Input: dimensioned drawing with shaded views. Units: mm. Origin: part minimum x, y, z. A direction names the side the tool comes from. Round coordinates to 2 decimals unless told otherwise and drop trailing zeros. Loops run counter-clockwise (first coordinate to the right, second up) from the corner with the lowest first, then second, coordinate; pieces in that order, holes last. Notation, with made-up numbers: (14.5, 26.5) - (27.5, 26.5) arc R21 cw to (27.5, 53.5) - close; hole circle Ø2 at (-20.75, -32.5). An arc over 180 degrees is marked (long way). One line per question, with ' | ' between items.
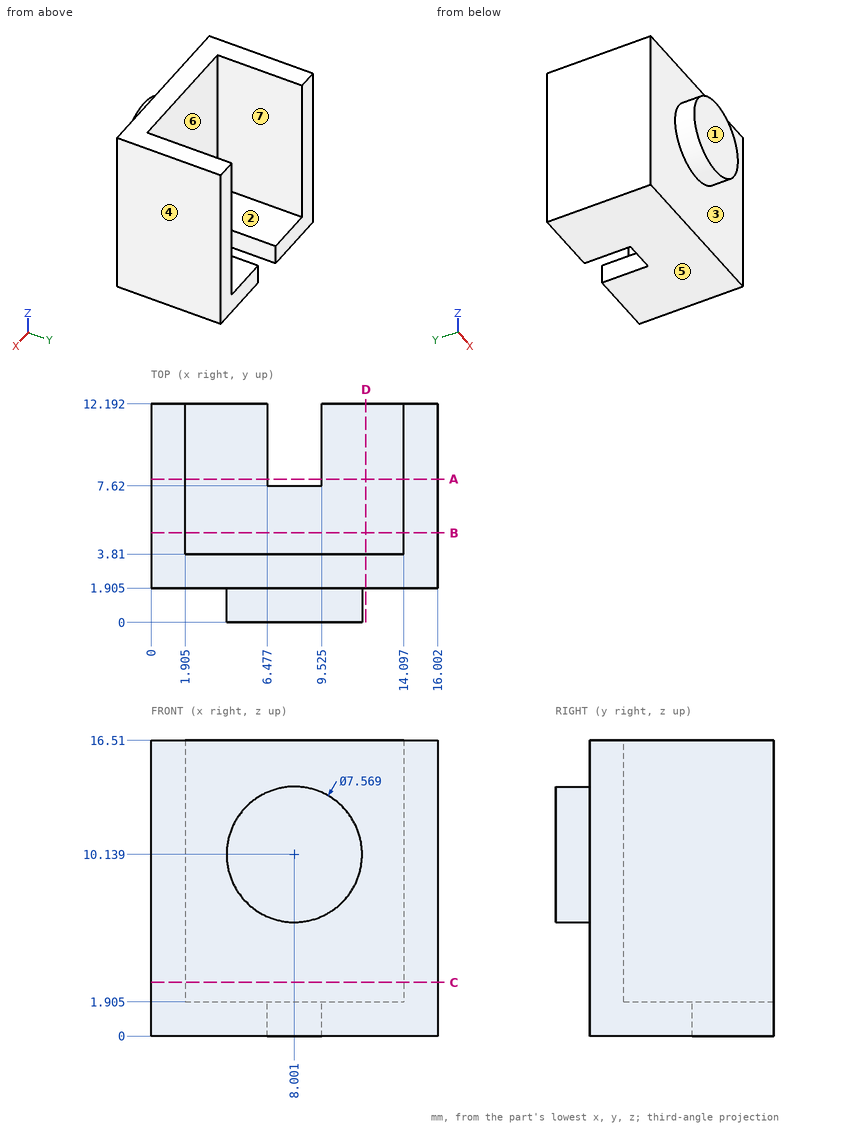
1. Material intervals for probe 1 along X at (y, z) = (9, 7) (1 decimal); probe 2 along Z at (x, y) = (5.5, 7) (1 decimal); probe 3 along Y at (x, z) = (5.5, 12.5), sorted ascending.
Worked out:
probe 1: x = 0 to 1.9, 14.1 to 16 | probe 2: z = 0 to 1.9 | probe 3: y = 0 to 3.81
2. Contact query for flat-ended pins moving along their axis: P1, Ø5, axis at x = 8, z = 8, coming from the +Y side; P2, Ø1.5, axis at x = 8.5, z = 1.5, coming from the +Y side; P3, Ø6.5, axis at x = 7, y = 9, coming from the +Z side (3 decimals). Output: stop coordinate, or through.
Worked out:
P1: stops at y = 3.81 | P2: stops at y = 7.62 | P3: stops at z = 1.905
3. Section query C-C, the plane z = 3. Return loops of the section in (x, y) (1 decimal).
Worked out:
outline: (0, 1.9) - (16, 1.9) - (16, 12.2) - (14.1, 12.2) - (14.1, 3.8) - (1.9, 3.8) - (1.9, 12.2) - (0, 12.2) - close
4. Access query for the marked faces 1, 2 and 3. Directions: +Z, -Z, +X, -X, +Y, -Y. A direction counts if a zero-diameter tool reaches every point of the face in a straight line with its end or side. Return the directions, or none.
Worked out:
face 1: +Z, -Z, +X, -X, -Y | face 2: +Z, +Y | face 3: -Y
5. Section query D-D, the plane x = 12. Return loops of the section in (y, z) (1 decimal).
Worked out:
outline: (1.9, 0) - (12.2, 0) - (12.2, 1.9) - (3.8, 1.9) - (3.8, 16.5) - (1.9, 16.5) - close
6. Section query B-B, the plane y = 5. Return loops of the section in (x, z) (1 decimal).
Worked out:
outline: (0, 0) - (16, 0) - (16, 16.5) - (14.1, 16.5) - (14.1, 1.9) - (1.9, 1.9) - (1.9, 16.5) - (0, 16.5) - close
7. Section query A-A, the plane y = 8. Return loops of the section in (x, z) (1 decimal).
Worked out:
outline: (0, 0) - (6.5, 0) - (6.5, 1.9) - (1.9, 1.9) - (1.9, 16.5) - (0, 16.5) - close; (9.5, 0) - (16, 0) - (16, 16.5) - (14.1, 16.5) - (14.1, 1.9) - (9.5, 1.9) - close
8. Mould query, pull axis X, two halves, no side actions, for the marked faces 4, 5, 6 and 7. Classes: released by +X, released by -X, zero draft, split by the parting line, or undercut.
Worked out:
face 4: released by +X | face 5: zero draft | face 6: undercut | face 7: undercut
